CAD build for the part. Positions are in the model's coordinates, mm. A direction names the side the tool comes from. Give positions to 0.01 mm unless a question says otherwise; leave off trailing zeros. Write each loop counter-clockwise with the first axis right and the second up, starting at its lowest first coordinate (ties: lowest second). Pieces come first, ordered by that corner, then holes. Notation, with made-up numbers: (34, 77) -> (52, 77) arc R31 ccw to (52, 104) -> close; hole circle Ø5 at (-27.75, 46.25). An arc over 180 degrees is marked (long way). Answer as a JSON object with one key per item and string values.
```python
from build123d import *

# Parameters (mm, degrees)
SKETCH1_W                 = 38.2
SKETCH1_H                 = 30
BOSS_EXTRUDE1_DEPTH       = 2
SKETCH2_W                 = 2
SKETCH2_H                 = 20
BOSS_EXTRUDE2_DEPTH       = 27.02
CUT_EXTRUDE1_REACH        = 58.632
SKETCH3_W                 = 7.09
SKETCH3_H                 = 23
CUT_EXTRUDE3_REACH        = 58.632
CUT_EXTRUDE4_DEPTH        = 57.632318808
CUT_EXTRUDE4_DEPTH_BACK   = 57.632318808
SKETCH7_W                 = 32.25
SKETCH7_H                 = 3
BOSS_EXTRUDE3_DEPTH       = 25.02
SKETCH8_W                 = 20
SKETCH8_H                 = 30
BOSS_EXTRUDE4_DEPTH       = 5
BOSS_EXTRUDE5_DEPTH       = 2
BOSS_EXTRUDE6_DEPTH       = 3
BOSS_EXTRUDE7_DEPTH       = 2
SKETCH12_W                = 5
SKETCH12_H                = 27.02
BOSS_EXTRUDE8_DEPTH       = 5
SKETCH13_W                = 5
SKETCH13_H                = 22
BOSS_EXTRUDE10_DEPTH      = 44
SKETCH15_W                = 5
SKETCH15_H                = 27.02
BOSS_EXTRUDE11_DEPTH      = 5
BOSS_EXTRUDE12_DEPTH      = 5.02
BOSS_EXTRUDE12_DEPTH_BACK = 2
SKETCH16_W                = 5
SKETCH16_H                = 44
SKETCH17_W                = 20
SKETCH17_H                = 34
CUT_EXTRUDE5_DEPTH        = 5


with BuildPart() as part:
    # Sketch1 → Boss-Extrude1 (new body)
    with BuildSketch(Plane.XY):
        with Locations((-9.254890621, -15.096829294)):
            Rectangle(SKETCH1_W, SKETCH1_H)
    extrude(amount=BOSS_EXTRUDE1_DEPTH)

    # Sketch2 → Boss-Extrude2 (add)
    with BuildSketch(Plane.XY.offset(2)):
        Polygon((-26.154890621, -2.096829294), (-28.354890621, -2.096829294), (-28.354890621, -30.096829294), (-26.154890621, -30.096829294), (-26.154890621, -22.146829294), (-27.154890621, -22.146829294), (-27.154890621, -7.046829294), (-26.154890621, -7.046829294), align=None)
        Polygon((9.845109379, -0.096829294), (-28.354890621, -0.096829294), (-28.354890621, -2.096829294), (-26.154890621, -2.096829294), (6.095109379, -2.096829294), (9.845109379, -2.096829294), align=None)
        Polygon((9.845109379, -4.596829294), (9.845109379, -2.096829294), (6.095109379, -2.096829294), (6.095109379, -4.596829294), (7.845109379, -4.596829294), align=None)
        with Locations((8.845109379, -14.596829294)):
            Rectangle(SKETCH2_W, SKETCH2_H)
        Polygon((9.845109379, -30.096829294), (9.845109379, -24.596829294), (7.845109379, -24.596829294), (6.095109379, -24.596829294), (6.095109379, -30.096829294), align=None)
    extrude(amount=BOSS_EXTRUDE2_DEPTH)

    # Sketch3 → Cut-Extrude1 (cut, up to next)
    with BuildSketch(Plane(origin=(9.845109379, 0, 0), x_dir=(0, 0, -1), z_dir=(1, 0, 0)), mode=Mode.PRIVATE) as cut_extrude1_sk1:
        with Locations((-25.475, -14.596829294)):
            Rectangle(SKETCH3_W, SKETCH3_H)
    cut_extrude1_tool1 = extrude(cut_extrude1_sk1.sketch, amount=-CUT_EXTRUDE1_REACH, mode=Mode.PRIVATE) & part.part
    add(cut_extrude1_tool1.solids().sort_by_distance((9.845109, -14.596829, 25.475))[0], mode=Mode.SUBTRACT)

    # Sketch4 → Cut-Extrude3 (cut, up to next)
    with BuildSketch(Plane.ZY.offset(28.354890621), mode=Mode.PRIVATE) as cut_extrude3_sk1:
        with BuildLine():
            ThreePointArc((25.02, -15.096829294), (26.063183829, -20.116789453), (29.02, -24.30552084))
            Line((29.02, -24.30552084), (29.02, -15.096829294))
            Line((29.02, -15.096829294), (25.02, -15.096829294))
        make_face()
    cut_extrude3_tool1 = extrude(cut_extrude3_sk1.sketch, amount=-CUT_EXTRUDE3_REACH, mode=Mode.PRIVATE) & part.part
    # Sketch4 → Cut-Extrude3 (cut, up to next)
    with BuildSketch(Plane.ZY.offset(28.354890621), mode=Mode.PRIVATE) as cut_extrude3_sk2:
        with BuildLine():
            ThreePointArc((29.02, -5.888137747), (26.063183829, -10.076869135), (25.02, -15.096829294))
            Line((25.02, -15.096829294), (29.02, -15.096829294))
            Line((29.02, -15.096829294), (29.02, -5.888137747))
        make_face()
    cut_extrude3_tool2 = extrude(cut_extrude3_sk2.sketch, amount=-CUT_EXTRUDE3_REACH, mode=Mode.PRIVATE) & part.part
    # Sketch4 → Cut-Extrude3 (cut, up to next)
    with BuildSketch(Plane.ZY.offset(28.354890621), mode=Mode.PRIVATE) as cut_extrude3_sk3:
        with BuildLine():
            ThreePointArc((25.02, -15.096829294), (26.063183829, -20.116789453), (29.02, -24.30552084))
            Line((29.02, -24.30552084), (29.02, -15.096829294))
            Line((29.02, -15.096829294), (25.02, -15.096829294))
        make_face()
    cut_extrude3_tool3 = extrude(cut_extrude3_sk3.sketch, amount=-CUT_EXTRUDE3_REACH, mode=Mode.PRIVATE) & part.part
    # Sketch4 → Cut-Extrude3 (cut, up to next)
    with BuildSketch(Plane.ZY.offset(28.354890621), mode=Mode.PRIVATE) as cut_extrude3_sk4:
        with BuildLine():
            ThreePointArc((29.02, -5.888137747), (26.063183829, -10.076869135), (25.02, -15.096829294))
            Line((25.02, -15.096829294), (29.02, -15.096829294))
            Line((29.02, -15.096829294), (29.02, -5.888137747))
        make_face()
    cut_extrude3_tool4 = extrude(cut_extrude3_sk4.sketch, amount=-CUT_EXTRUDE3_REACH, mode=Mode.PRIVATE) & part.part
    add(cut_extrude3_tool1.solids().sort_by_distance((-28.354891, -18.637073, 27.396015))[0], mode=Mode.SUBTRACT)
    add(cut_extrude3_tool2.solids().sort_by_distance((-28.354891, -11.556586, 27.396015))[0], mode=Mode.SUBTRACT)
    add(cut_extrude3_tool3.solids().sort_by_distance((-28.354891, -18.637073, 27.396015))[0], mode=Mode.SUBTRACT)
    add(cut_extrude3_tool4.solids().sort_by_distance((-28.354891, -11.556586, 27.396015))[0], mode=Mode.SUBTRACT)

    # Sketch6 → Cut-Extrude4 (cut, two sides: drawn at the far end of the back side and taken through both)
    with BuildSketch(Plane.ZY.offset(28.354890621).offset(-CUT_EXTRUDE4_DEPTH_BACK)):
        with BuildLine():
            Line((29.02, -30.096829294), (29.02, -24.30552084))
            ThreePointArc((29.02, -24.30552084), (27.945480542, -23.169231244), (27.02, -21.90858384))
            Line((27.02, -21.90858384), (27.02, -30.096829294))
            Line((27.02, -30.096829294), (29.02, -30.096829294))
        make_face()
        with BuildLine():
            Line((29.02, -5.888137747), (29.02, -0.096829294))
            Line((29.02, -0.096829294), (27.02, -0.096829294))
            Line((27.02, -0.096829294), (27.02, -8.285074747))
            ThreePointArc((27.02, -8.285074747), (27.945480542, -7.024427343), (29.02, -5.888137747))
        make_face()
    extrude(amount=CUT_EXTRUDE4_DEPTH + CUT_EXTRUDE4_DEPTH_BACK, mode=Mode.SUBTRACT)

    # Sketch7 → Boss-Extrude3 (add)
    with BuildSketch(Plane.XY.offset(2)):
        with Locations((-10.029890621, -28.596829294)):
            Rectangle(SKETCH7_W, SKETCH7_H)
    extrude(amount=BOSS_EXTRUDE3_DEPTH)

    # Sketch8 → Boss-Extrude4 (add)
    with BuildSketch(Plane.ZY.offset(28.354890621)):
        with Locations((10, -15.096829294)):
            Rectangle(SKETCH8_W, SKETCH8_H)
    extrude(amount=BOSS_EXTRUDE4_DEPTH)

    # Sketch9 → Boss-Extrude5 (add)
    with BuildSketch(Plane.XZ.offset(30.096829294)):
        Polygon((-33.354890621, 20), (-28.354890621, 20), (-28.354890621, 27.02), (9.845109379, 27.02), (9.845109379, 0), (-33.354890621, 0), align=None)
    extrude(amount=BOSS_EXTRUDE5_DEPTH)

    # Sketch10 → Boss-Extrude6 (add)
    with BuildSketch(Plane(origin=(9.845109379, 0, 0), x_dir=(0, 0, -1), z_dir=(1, 0, 0))):
        Polygon((-21.93, -3.096829294), (-21.93, -26.096829294), (-27.02, -26.096829294), (-27.02, -32.096829294), (0, -32.096829294), (0, -0.096829294), (-27.02, -0.096829294), (-27.02, -3.096829294), align=None)
    extrude(amount=BOSS_EXTRUDE6_DEPTH)

    # Sketch11 → Boss-Extrude7 (add)
    with BuildSketch(Plane(origin=(0, -0.096829294, 0), x_dir=(1, 0, 0), z_dir=(0, 1, 0))):
        Polygon((-33.354890621, 0), (-33.354890621, -20), (-28.354890621, -20), (-28.354890621, -27.02), (12.845109379, -27.02), (12.845109379, 0), align=None)
    extrude(amount=BOSS_EXTRUDE7_DEPTH)

    # Sketch12 → Boss-Extrude8 (add)
    with BuildSketch(Plane(origin=(0, 1.903170706, 0), x_dir=(1, 0, 0), z_dir=(0, 1, 0))):
        with Locations((5.345109379, -13.51)):
            Rectangle(SKETCH12_W, SKETCH12_H)
    extrude(amount=BOSS_EXTRUDE8_DEPTH)

    # Sketch13 → Boss-Extrude10 (add)
    with BuildSketch(Plane(origin=(0, 6.903170706, 0), x_dir=(1, 0, 0), z_dir=(0, 1, 0))):
        with Locations((15.345109379, -11)):
            Rectangle(SKETCH13_W, SKETCH13_H)
    extrude(amount=-BOSS_EXTRUDE10_DEPTH)

    # Sketch15 → Boss-Extrude11 (add)
    with BuildSketch(Plane(origin=(0, -32.096829294, 0), x_dir=(-1, 0, 0), z_dir=(0, -1, 0))):
        with Locations((-5.345109379, -13.51)):
            Rectangle(SKETCH15_W, SKETCH15_H)
    extrude(amount=BOSS_EXTRUDE11_DEPTH)

    # Sketch16 → Boss-Extrude12 (add, two sides: drawn at the far end of the back side and taken through both)
    with BuildSketch(Plane.XY.offset(22).offset(-BOSS_EXTRUDE12_DEPTH_BACK)):
        with Locations((15.345109379, -15.096829294)):
            Rectangle(SKETCH16_W, SKETCH16_H)
    extrude(amount=BOSS_EXTRUDE12_DEPTH + BOSS_EXTRUDE12_DEPTH_BACK)

    # Sketch17 → Cut-Extrude5 (cut)
    with BuildSketch(Plane.ZY.offset(33.354890621)):
        with Locations((10, -15.096829294)):
            Rectangle(SKETCH17_W, SKETCH17_H)
    extrude(amount=-CUT_EXTRUDE5_DEPTH, mode=Mode.SUBTRACT)


solid = part.part
```
1) Slice it at C-C (x = 10). List the corners of the cut face in (y, z).
Model answer:
{"outline": "(-32.1, 0) -> (1.9, 0) -> (1.9, 27.02) -> (-3.1, 27.02) -> (-3.1, 21.93) -> (-26.1, 21.93) -> (-26.1, 27.02) -> (-32.1, 27.02) -> close"}
2) Wall check: probe 1 along Y at (x, z) = (-20, 6.5); probe 2 along X at (y, z) = (-25, 17.25); probe 3 along X at (y, z) = (-23, 6.25). Give the ranges that are in metal, low to high.
Model answer:
{"probe 1": "y = -32.1 to -27.1, -2.1 to 1.9", "probe 2": "x = -28.35 to -26.15, 6.1 to 17.85", "probe 3": "x = -28.35 to -26.15, 7.85 to 17.85"}
3) 3-axis set-ups, long thin cutter, end or side, ignore diameter. For faces 4 (the flat face through (-10, -27.097, 14)), 5 (the flat face through (2.845, 4, 14)), 6 (the flat face through (10, 1.903, 13)), 7 (the flat face through (10, -32.097, 14)): which of +Z, -Z, +X, -X, +Y, -Y reach the whole face in a straight line?
Model answer:
{"face 4": "+Z", "face 5": "+Z, -Z, -X, +Y", "face 6": "+Z, -Z, +Y", "face 7": "+Z, -Z, -Y"}
4) Mould opens along Y. For faces 1 (the flat face through (-10, -2.097, 14)), 2 (the flat face through (-6, -15, 0)), 3 (the flat face through (-13, 1.903, 13)) say: released by +Y, released by -Y, zero draft, split by the parting line, or undercut.
Model answer:
{"face 1": "undercut", "face 2": "zero draft", "face 3": "released by +Y"}
5) Slice it at A-A (y = -34). List the corners of the cut face in (x, z).
Model answer:
{"outline": "(2.85, 0) -> (7.85, 0) -> (7.85, 27.02) -> (2.85, 27.02) -> close; (12.85, 0) -> (17.85, 0) -> (17.85, 27.02) -> (12.85, 27.02) -> close"}
6) Pin check, flat tips, straight feed: pin 1 (2.5 mm diameter, centred on y = -34.5, z = 13.5, fed in from -X); pin 2 (8 mm diameter, centred on x = -13, z = 7, fed in from +Y); pin 3 (20 mm diameter, centred on x = -3, y = -16, fed in from +Z). Stop position of each tip, or through.
Model answer:
{"pin 1": "stops at x = 2.85", "pin 2": "stops at y = 1.9", "pin 3": "stops at z = 2"}
7) Slice it at B-B (z = 9.75). List the corners of the cut face in (x, y), then the cut area to 3 significant figures.
Model answer:
{"outline": "(-28.35, -32.1) -> (2.85, -32.1) -> (2.85, -37.1) -> (7.85, -37.1) -> (7.85, -32.1) -> (12.85, -32.1) -> (12.85, -37.1) -> (17.85, -37.1) -> (17.85, 6.9) -> (12.85, 6.9) -> (12.85, 1.9) -> (7.85, 1.9) -> (7.85, 6.9) -> (2.85, 6.9) -> (2.85, 1.9) -> (-28.35, 1.9) -> close; hole (-27.15, -22.15) -> (-26.15, -22.15) -> (-26.15, -27.1) -> (6.1, -27.1) -> (6.1, -24.6) -> (7.85, -24.6) -> (7.85, -4.6) -> (6.1, -4.6) -> (6.1, -2.1) -> (-26.15, -2.1) -> (-26.15, -7.05) -> (-27.15, -7.05) -> close", "area": "814 mm2"}
8) Slice it at D-D (y = -23). List the corners of the cut face in (x, z), then the cut area to 3 significant figures.
Model answer:
{"outline": "(-28.35, 0) -> (17.85, 0) -> (17.85, 27.02) -> (12.85, 27.02) -> (12.85, 21.93) -> (7.85, 21.93) -> (7.85, 2) -> (-26.15, 2) -> (-26.15, 27.02) -> (-28.35, 27.02) -> close", "area": "372 mm2"}
